Part model, mm, in its own coordinate system. A direction names the side the tool comes from. Round coordinates to 2 decimals unless told otherwise and drop trailing zeros. Loops run counter-clockwise (first coordinate to the right, second up) from the corner with the lowest first, then second, coordinate; pieces in that order, holes last.
1) 3-axis set-ups, long thin cutter, end or side, ignore diameter. For faces 1 (the flat face through (-20, 19, 25)), 2 (the flat face through (-8, -12, 6.857)), 3 (the flat face through (-15.181, -12, 16)): which of +Z, -Z, +X, -X, +Y, -Y reach the whole face in a straight line?
2) Drop flat-ended pins along their axis: P1, Ø4, axis at x = 13, y = -10, coming from the -Z side; P2, Ø4, axis at y = -2, z = 7, coming from the +X side; P3, Ø5, axis at y = -14, z = 21.5, coming from the -X side. Give the stop position or say it passes through.
3) Band-saw the part on A-A, the plane x = -3. Write the cut outline in (y, z), then the cut area to 3 significant figures.
4) Band-saw the part on B-B, the plane z = 12. Write the cut outline in (x, y), then the cut area to 3 significant figures.
5) Band-saw the part on C-C, the plane y = 4.5. Write the cut outline in (x, z).
6) Probe line 1 (Y direction, x = -30, z = 13.75); line 2 (X direction, y = 32, z = 13.25); line 3 (X direction, y = -3, z = 7.75). List the from-to ranges inside material, lowest first.
7) Band-saw the part on D-D, the plane x = -33.5. Write the cut outline in (y, z), then the cut area to 3 significant figures.
from build123d import *

# Parameters (mm, degrees)
F0_W     = 38.61342
F0_H     = 37.553012
F1_DEPTH = 25
F2_W     = 15.180568
F2_H     = 18.142793
F3_DEPTH = 25
F4_R     = 7.086632
F5_ANGLE = 90


with BuildPart() as f1:
    # F0 (on Top) → F1 (new body)
    with BuildSketch(Plane.XY):
        with Locations((-19.30671, 18.776506)):
            Rectangle(F0_W, F0_H)
    extrude(amount=F1_DEPTH)

    # F2 (on face) → F3 (join)
    with BuildSketch(Plane.XZ):
        with Locations((-7.590284, 15.928603)):
            Rectangle(F2_W, F2_H)
    extrude(amount=F3_DEPTH)

    # F4 (on face) → F5 (revolve)
    with BuildSketch(Plane.YZ):
        with Locations((-12.13547, 16.139457)):
            Circle(F4_R)
    revolve(axis=Axis((0, -25, 15.928603), (0, 0, -1)), revolution_arc=F5_ANGLE)


solid = f1.part
Reported:
1. face 1: +Z, +X, -X, +Y, -Y
1. face 2: -Z, +X, -X, -Y
1. face 3: +Z, -Z, -X, -Y
2. P1: stops at z = 11.1
2. P2: stops at x = 0
2. P3: stops at x = -15.18
3. outline: (-25, 6.86) - (0, 6.86) - (0, 0) - (37.55, 0) - (37.55, 25) - (-25, 25) - close
3. area: 1,390 mm2
4. outline: (-38.61, 0) - (-15.18, 0) - (-15.18, -25) - (0, -25) - (0, -17.89) arc R7.11 cw to (7.11, -25) - (18.62, -25) arc R18.62 ccw to (0, -6.38) - (0, 37.55) - (-38.61, 37.55) - close
4. area: 2,060 mm2
5. outline: (-38.61, 0) - (0, 0) - (0, 25) - (-38.61, 25) - close
6. line 1: y = 0 to 37.55
6. line 2: x = -38.61 to 0
6. line 3: x = -15.18 to 0
7. outline: (0, 0) - (37.55, 0) - (37.55, 25) - (0, 25) - close
7. area: 939 mm2
